from build123d import *

# Parameters (mm, degrees)
SKETCH_1_R      = 1.525
EXTRUDE_1_DEPTH = 2
FILLET_1_R      = 3


with BuildPart() as part:
    # 草图1 → 凸台-拉伸1 (new body)
    with BuildSketch(Plane(origin=(0, 0, 0), x_dir=(1, 0, 0), z_dir=(0, 1, 0))):
        Polygon((-5, 30), (5, 30), (25, 10), (25, 0), (-25, 0), (-25, 10), align=None)
        with Locations(Location((0, 25, 0), (0, 0, 270))):
            Circle(SKETCH_1_R, mode=Mode.SUBTRACT)
        with Locations(Location((0, 15, 0), (0, 0, 270))):
            Circle(SKETCH_1_R, mode=Mode.SUBTRACT)
        with Locations(Location((0, 5, 0), (0, 0, 270))):
            Circle(SKETCH_1_R, mode=Mode.SUBTRACT)
        with Locations(Location((10, 5, 0), (0, 0, 270))):
            Circle(SKETCH_1_R, mode=Mode.SUBTRACT)
        with Locations(Location((-10, 5, 0), (0, 0, 270))):
            Circle(SKETCH_1_R, mode=Mode.SUBTRACT)
        with Locations(Location((20, 5, 0), (0, 0, 270))):
            Circle(SKETCH_1_R, mode=Mode.SUBTRACT)
        with Locations(Location((-20, 5, 0), (0, 0, 270))):
            Circle(SKETCH_1_R, mode=Mode.SUBTRACT)
    extrude(amount=EXTRUDE_1_DEPTH)

    # 圆角1
    fillet_1_edges = [part.edges().sort_by_distance(p)[0] for p in [
        (-5, 1, -30),
        (5, 1, -30),
        (25, 1, -10),
        (25, 1, 0),
        (-25, 1, 0),
        (-25, 1, -10),
    ]]
    fillet(fillet_1_edges, radius=FILLET_1_R)


solid = part.part
CAD build for the part. Positions are in the model's coordinates, mm. Give positions to 0.01 mm unless a question says otherwise; leave off trailing zeros. Write each loop counter-clockwise with the first axis right and the second up, starting at its lowest first coordinate (ties: lowest second). Pieces come first, ordered by that corner, then holes. Notation, with made-up numbers: (-4, 68.25) - (21, 68.25) arc R13 ccw to (21, 73.25) - close; hole circle Ø7 at (60, -35). An arc over 180 degrees is marked (long way). Put each result on its own line as item: value.
(1) Saw through at B-B (z = -5). List the corners of the cut face in (x, y) (3 decimals), then the cut area to 3 significant figures.
Working result:
outline: (-25, 0) - (-21.525, 0) - (-21.525, 2) - (-25, 2) - close; (-18.475, 0) - (-11.525, 0) - (-11.525, 2) - (-18.475, 2) - close; (-8.475, 0) - (-1.525, 0) - (-1.525, 2) - (-8.475, 2) - close; (1.525, 0) - (8.475, 0) - (8.475, 2) - (1.525, 2) - close; (11.525, 0) - (18.475, 0) - (18.475, 2) - (11.525, 2) - close; (21.525, 0) - (25, 0) - (25, 2) - (21.525, 2) - close
area: 69.5 mm^2
(2) Pull direction Z, two halves, no side cores. Call faces 1 (the cylindrical face through (24.765, 1.014, -9.921)), 2 (the cylindrical face through (-24.14, 1.01, -0.9)), 3 (the cylindrical face through (-0.6, 1, -13.6)), 4 (the flat face through (0, 2, -12)): released by +Z, released by -Z, zero draft, split by the parting line, or undercut.
Working result:
face 1: released by -Z
face 2: released by +Z
face 3: undercut
face 4: zero draft
(3) Saw through at C-C (x = 0). List the corners of the cut face in (y, z) (3 decimals), then the cut area to 3 significant figures.
Working result:
outline: (0, -30) - (2, -30) - (2, -26.525) - (0, -26.525) - close; (0, -23.475) - (2, -23.475) - (2, -16.525) - (0, -16.525) - close; (0, -13.475) - (2, -13.475) - (2, -6.525) - (0, -6.525) - close; (0, -3.475) - (2, -3.475) - (2, 0) - (0, 0) - close
area: 41.7 mm^2
(4) Wall check: L1, parallel to X at y = 0.9, z = -5 (3 decimals); L2, parallel to Z at x = -20.5, y = 1; L3, parallel to Z at x = -13, y = 1.55. Give the ranges that are in metal, low to high.
Working result:
L1: -25 to -21.525, -18.475 to -11.525, -8.475 to -1.525, 1.525 to 8.475, 11.525 to 18.475, 21.525 to 25
L2: -14.5 to -6.44, -3.56 to 0
L3: -22 to 0
(5) Saw through at D-D (z = -15). List the corners of the cut face in (x, y) (3 decimals), then the cut area to 3 significant figures.
Working result:
outline: (-20, 0) - (-1.525, 0) - (-1.525, 2) - (-20, 2) - close; (1.525, 0) - (20, 0) - (20, 2) - (1.525, 2) - close
area: 73.9 mm^2
(6) Saw through at A-A (x = 10). List the corners of the cut face in (y, z) (3 decimals), then the cut area to 3 significant figures.
Working result:
outline: (0, -25) - (2, -25) - (2, -6.525) - (0, -6.525) - close; (0, -3.475) - (2, -3.475) - (2, 0) - (0, 0) - close
area: 43.9 mm^2
